Verification items for the finished model (mm, model axes). Face numbers are marked on the shaded views. Coordinates: 2 decimals unless noted, no trailing zeros. Write each loop counter-clockwise with the first axis right and the second up, starting at its lowest first coordinate (ties: lowest second). Pieces come first, ordered by that corner, then holes. Notation, with made-up numbers: (-15.75, 86) -> (7.25, 86) arc R10 ccw to (7.25, 103) -> close; hole circle Ø2 at (65.5, 22.25). An arc over 180 degrees is marked (long way). Write each question's results on one line, items separated by ' | '. Start each with the question number.
Autodesk Inventor part; units mm, degrees
ref_plane "Work Plane1" through (1.525, 0, 0) normal (0, 0, 1) x (1, 0, 0)
ref_plane "YZ Plane" through (0, 0, 0) normal (1, 0, 0) x (0, 1, 0)
ref_plane "XZ Plane" through (0, 0, 0) normal (0, 1, 0) x (-1, 0, 0)
sketch "Sketch1" plane through (0, 0, 0) normal (0, 0, 1) x (1, 0, 0)
  line L0 (0, 5.5626) -> (0, 3.175)
  line L1 (95.25, 3.175) -> (114.3, 3.175)
  line L2 (114.3, 3.175) -> (114.3, 0)
  line L3 (114.3, 0) -> (-0.6351, 0)
  line L4 (-23.6221, 0) -> (137.287, 0)
  line L5 (-0.6351, 0) -> (-0.6351, 5.5626)
  line L6 (-0.6351, 5.5626) -> (0, 5.5626)
  line L7 (95.25, 3.175) -> (85.0899, 3.175)
  line L8 (85.0899, 3.175) -> (0, 3.175)
  line L9 (0, -1.1125) -> (0, 6.6751)
  dimension "d0" = 114.3
  dimension "d1" = 19.05
  dimension "d2" = 6.35
  dimension "d9" = 0.6351
  dimension "d10" = 11.1252
  dimension "d13" = 10.1601
  dimension "d14" = 6.35
revolve "Body" add sketch "Sketch1" angle 360 about axis through (114.3, 0, 0) along (-1, 0, 0)
sketch "Sketch2" plane through (-0.6351, 0, 0) normal (-1, 0, 0) x (0, 0, 1)
  line L0 (0, 6.4231) -> (5.5626, 3.2116)
  line L1 (5.5626, 3.2116) -> (5.5626, -3.2116)
  line L2 (5.5626, -3.2116) -> (0, -6.4231)
  line L3 (0, -6.4231) -> (-5.5626, -3.2116)
  line L4 (-5.5626, -3.2116) -> (-5.5626, 3.2116)
  line L5 (-5.5626, 3.2116) -> (0, 6.4231)
  point P0 (0, 0)
  point P1 (0, 0)
  dimension "d11" = 11.1252
extrude "Head" add sketch "Sketch2" along normal blind 3.5052
sketch "Sketch4" plane through (0, 0, 0) normal (0, 0, 1) x (1, 0, 0)
  line L0 (-4.1403, 5.5626) -> (-4.1403, 6.4231)
  line L1 (-4.1403, 6.4231) -> (-3.6435, 6.4231)
  line L2 (-3.6435, 6.4231) -> (-4.1403, 5.5626)
  line L3 (-4.8413, 0) -> (0.0659, 0)
  line L4 (-0.6351, 6.4231) -> (-4.1403, 6.4231)
  line L5 (-4.1403, 3.2116) -> (-4.1403, 6.4231)
  dimension "d5" = 30
  dimension "d19" = 11.1252
revolve "Chamfer1" cut sketch "Sketch4" angle 360 about axis through (-10, 0, 0) along (1, 0, 0)
thread "Thread"
chamfer "Chamfer2" distance 0.779 distance2 0.7791 1 edges at (114.3, -3.175, 0) measured on face at (114.3, 0.6107, -1.4381)
ref_plane "Work Plane1" through (1.525, 0, 0) normal (0, 0, 1) x (1, 0, 0)
equation "\"d0\" = NLG"
equation "\"d1\" = GEL"
equation "\"d2\" = GD"
equation "\"d10\" = SD2"
equation "\"d14\" = BDM"
equation "\"d11\" = SW"
equation "\"d3\" = KOH - SD"
equation "\"d5\" = ANG1"
equation "\"d19\" = SW0"
equation "\"d15\" = GEL"
equation "\"d6\" = -0.5 * SPD + 0.5 * GD"
equation "\"NLG\" = 114.3"
equation "\"GD\" = 6.35"
equation "\"BDM\" = 6.35"
equation "\"KOH\" = 4.1402"
equation "\"GEL\" = 19.05"
equation "\"SW\" = 11.1252"
equation "\"SW0\" = SW"
equation "\"SPD\" = GD1"
equation "\"SD2\" = SW"
equation "\"SD\" = 0.635"
equation "\"ANG1\" = 30deg"
equation "\"GAL\" = 10.16"
equation "\"GUL\" = 0.77902"
equation "\"RR\" = 0.381"
equation "\"WFT\" = SD"
equation "\"GD1\" = 4.79196"
equation "\"THREADDIA\" = 6.35"
equation "\"SDH\" = SW"
equation "\"SDHG\" = 85.09"
equation "\"TOA\" = 30deg"
equation "\"FAWI\" = 45deg"
equation "\"NND\" = 6.35"
equation "\"E0\" = 12.84961"
properties part number "AS 2465 - 1/4 x 4 1/2  UNC" material "Steel, Mild"
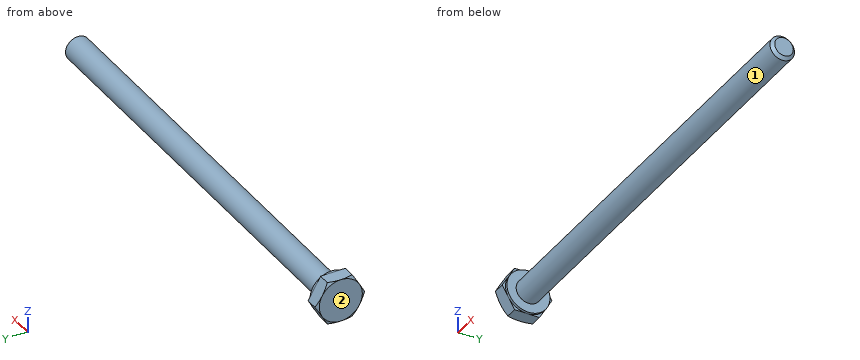
1. Depth check by flat-ended pin: pin 1 Ø4 at (y, z) = (3.5, 1) entering from +X; pin 2 Ø0.8 at (y, z) = (-2, 4) entering from +X; pin 3 Ø1 at (x, z) = (22.5, 3) entering from -Y; pin 4 Ø1 at (x, y) = (42.5, 2.5) entering from -Z. Enter the tip coordinate at first touch or a pass-through.
2. Material ranges on probe 1 along Y at (x, z) = (49.5, 0) (3 decimals); probe 2 along Z at (x, y) = (29, 0.25); probe 3 along Y at (x, z) = (28, 1.5), recorded low to high. Write a range as from..to.
3. Mould release check, pull along Y, two halves, no side actions. Record for the marked faces 1 and 2: +Y half, -Y half, draft (parallel to the pull), parting line (faces both ways), or undercut.
4. Sectioned sample at A-A on x = 102.5. Record the cut outline in (y, z) (3 decimals), plus the area to 3 significant figures.
Computed values:
1) pin 1: stops at x = 114.3 | pin 2: stops at x = 0 | pin 3: stops at y = -1.96 | pin 4: stops at z = -2.47
2) probe 1: y = -3.175..3.175 | probe 2: z = -3.17..3.17 | probe 3: y = -2.8..2.8
3) face 1: parting line | face 2: draft
4) outline: circle Ø6.35 at (0, 0) | area: 31.7 mm^2
